The listing builds one solid part. Answer for the finished solid, in the listing's coordinates (mm). A direction names the side the tool comes from. Coordinates: 2 decimals unless noted, no trailing zeros. Order: outer loops, then holes, each group sorted by start corner. A loop starts at its lowest first (then second) coordinate and runs counter-clockwise, first axis right, second up.
from build123d import *

# Parameters (mm, degrees)
EXTRUDE_2_DEPTH      = 10
SKETCH_6_R           = 2.5
CUT_EXTRUDE_1_DEPTH  = 8
SKETCH_7_R           = 5.5
CUT_EXTRUDE_2_DEPTH  = 114.578166916
CUT_EXTRUDE_3_DEPTH  = 114.578166916
CUT_EXTRUDE_4_DEPTH  = 3
FILLET_1_R           = 2
CUT_EXTRUDE_7_DEPTH  = 114.578166916
SKETCH_16_R          = 3.5
CUT_EXTRUDE_8_DEPTH  = 3
SKETCH_18_R          = 2.1
CUT_EXTRUDE_9_DEPTH  = 114.578166916
FILLET_2_R           = 20
FILLET_3_R           = 2.5
SKETCH_20_R          = 3.75
CUT_EXTRUDE_11_DEPTH = 3
SKETCH_21_R          = 2.25
CUT_EXTRUDE_12_DEPTH = 114.578166916
SKETCH_22_R          = 7.1
CUT_EXTRUDE_13_DEPTH = 114.578166916


with BuildPart() as part:
    # 草图5 → 凸台-拉伸2 (new body)
    with BuildSketch(Plane.XY):
        with BuildLine():
            Line((-67.5, 42.938910093), (67.5, 42.938910093))
            ThreePointArc((67.5, 42.938910093), (0, -80), (-67.5, 42.938910093))
        make_face()
    extrude(amount=EXTRUDE_2_DEPTH)

    # 草图6 → 切除-拉伸1 (cut)
    with BuildSketch(Plane(origin=(0, 0, 0), x_dir=(-1, 0, 0), z_dir=(0, 0, -1))):
        with Locations(Location((-51.961524227, 30, 0), (0, 0, 180))):
            Circle(SKETCH_6_R)
        with Locations((-51.961524227, -30)):
            Circle(SKETCH_6_R)
        with Locations((51.961524227, -30)):
            Circle(SKETCH_6_R)
        with Locations(Location((51.961524227, 30, 0), (0, 0, 180))):
            Circle(SKETCH_6_R)
    extrude(amount=-CUT_EXTRUDE_1_DEPTH, mode=Mode.SUBTRACT)

    # 草图7 → 切除-拉伸2 (cut, through all)
    with BuildSketch(Plane(origin=(0, 0, 0), x_dir=(-1, 0, 0), z_dir=(0, 0, -1))):
        with Locations((32.939911054, -27.639867217)):
            Circle(SKETCH_7_R)
        with Locations((32.939911054, 27.639867217)):
            Circle(SKETCH_7_R)
        with Locations((-32.946514438, 27.631995701)):
            Circle(SKETCH_7_R)
        with Locations((-32.946514438, -27.631995701)):
            Circle(SKETCH_7_R)
    extrude(amount=-CUT_EXTRUDE_2_DEPTH, mode=Mode.SUBTRACT)

    # 草图8 → 切除-拉伸3 (cut, through all)
    with BuildSketch(Plane.XY.offset(10)):
        with BuildLine():
            ThreePointArc((-9.2723103, -65.975915967), (0, -66.624299065), (9.2723103, -65.975915967))
            ThreePointArc((9.2723103, -65.975915967), (14.814767997, -58.620826181), (7.459678211, -53.078368485))
            ThreePointArc((7.459678211, -53.078368485), (0, -53.6), (-7.459678211, -53.078368485))
            ThreePointArc((-7.459678211, -53.078368485), (-14.814767997, -58.620826181), (-9.2723103, -65.975915967))
        make_face()
    extrude(amount=-CUT_EXTRUDE_3_DEPTH, mode=Mode.SUBTRACT)

    # 草图9 → 切除-拉伸4 (cut)
    with BuildSketch(Plane.XY.offset(10)):
        with BuildLine():
            Line((-35.246116648, 34.895820279), (-25.683957992, 25.333661623))
            ThreePointArc((-25.683957992, 25.333661623), (-25.683957992, 20.383914155), (-30.63370546, 20.383914155))
            Line((-30.63370546, 20.383914155), (-40.195864116, 29.94607281))
            ThreePointArc((-40.195864116, 29.94607281), (-40.195864116, 34.895820279), (-35.246116648, 34.895820279))
        make_face()
        with BuildLine():
            Line((39.832192061, 29.567925856), (31.010584282, 20.746318078))
            ThreePointArc((31.010584282, 20.746318078), (26.060836814, 20.746318078), (26.060836814, 25.696065546))
            Line((26.060836814, 25.696065546), (34.882444593, 34.517673324))
            ThreePointArc((34.882444593, 34.517673324), (39.832192061, 34.517673324), (39.832192061, 29.567925856))
        make_face()
        with BuildLine():
            Line((-35.246116648, -34.895820279), (-25.683957992, -25.333661623))
            ThreePointArc((-25.683957992, -25.333661623), (-25.683957992, -20.383914155), (-30.63370546, -20.383914155))
            Line((-30.63370546, -20.383914155), (-40.195864116, -29.94607281))
            ThreePointArc((-40.195864116, -29.94607281), (-40.195864116, -34.895820279), (-35.246116648, -34.895820279))
        make_face()
        with BuildLine():
            Line((39.832192061, -29.567925856), (31.010584282, -20.746318078))
            ThreePointArc((31.010584282, -20.746318078), (26.060836814, -20.746318078), (26.060836814, -25.696065546))
            Line((26.060836814, -25.696065546), (34.882444593, -34.517673324))
            ThreePointArc((34.882444593, -34.517673324), (39.832192061, -34.517673324), (39.832192061, -29.567925856))
        make_face()
    extrude(amount=-CUT_EXTRUDE_4_DEPTH, mode=Mode.SUBTRACT)

    # 圆角1
    # the kernel refuses this fillet: 2 mm, written as the material it takes off along each edge
    with BuildSketch(Plane(origin=(32.421388172, -22.157121967, 12.140947066), x_dir=(0.9995822889813627, 0.028900649729367227, 0), z_dir=(0, 0, -1)), Plane(origin=(33.471640703, -33.106869435, 12.140947066), x_dir=(-0.9995822889813627, -0.028900649729367227, 0), z_dir=(0, 0, -1)), Plane(origin=(38.421388172, 28.157121967, 12.140947066), x_dir=(0.028900649729366526, -0.9995822889813627, 0), z_dir=(0, 0, -1)), Plane(origin=(27.471640703, 27.106869435, 12.140947066), x_dir=(-0.028900649729366384, 0.9995822889813627, 0), z_dir=(0, 0, -1)), Plane(origin=(-33.46503732, 33.114740951, 12.140947066), x_dir=(0.9995822889813627, 0.028900649729368344, 0), z_dir=(0, 0, -1)), Plane(origin=(-32.414784788, 22.164993482, 12.140947066), x_dir=(-0.9995822889813627, -0.028900649729368344, 0), z_dir=(0, 0, -1)), Plane(origin=(-27.46503732, -27.114740951, 12.140947066), x_dir=(0.028900649729362526, -0.9995822889813628, 0), z_dir=(0, 0, -1)), Plane(origin=(-38.414784788, -28.164993482, 12.140947066), x_dir=(-0.028900649729357547, 0.9995822889813629, 0), z_dir=(0, 0, -1))) as fillet_1_piece_1:
        with BuildLine():
            CenterArc((0.866697016, -1.995550294), FILLET_1_R, 93.822687788, 42.833428066)
            Line((-0.587797505, -0.622799155), (0, 0))
            ThreePointArc((0, 0), (0.366679507, -0.012236691), (0.733359013, 0))
        make_face()
    extrude(amount=5.140947066, mode=Mode.SUBTRACT)
    with BuildSketch(Plane(origin=(27.471640703, -27.106869435, 12.140947066), x_dir=(-0.028900649729367366, -0.9995822889813627, 0), z_dir=(0, 0, -1)), Plane(origin=(38.421388172, -28.157121967, 12.140947066), x_dir=(0.028900649729367924, 0.9995822889813627, 0), z_dir=(0, 0, -1)), Plane(origin=(33.471640703, 33.106869435, 12.140947066), x_dir=(-0.9995822889813627, 0.028900649729367227, 0), z_dir=(0, 0, -1)), Plane(origin=(32.421388172, 22.157121967, 12.140947066), x_dir=(0.9995822889813627, -0.028900649729367227, 0), z_dir=(0, 0, -1)), Plane(origin=(-38.414784788, 28.164993482, 12.140947066), x_dir=(-0.028900649729367647, -0.9995822889813627, 0), z_dir=(0, 0, -1)), Plane(origin=(-27.46503732, 27.114740951, 12.140947066), x_dir=(0.028900649729362664, 0.9995822889813628, 0), z_dir=(0, 0, -1)), Plane(origin=(-32.414784788, -22.164993482, 12.140947066), x_dir=(-0.9995822889813627, 0.028900649729368066, 0), z_dir=(0, 0, -1)), Plane(origin=(-33.46503732, -33.114740951, 12.140947066), x_dir=(0.9995822889813627, -0.028900649729367785, 0), z_dir=(0, 0, -1))) as fillet_1_piece_2:
        with BuildLine():
            CenterArc((0.866697016, 1.995550294), FILLET_1_R, 223.343884146, 42.833428066)
            Line((-0.587797505, 0.622799155), (0, 0))
            ThreePointArc((0, 0), (0.366679507, 0.012236691), (0.733359013, 0))
        make_face()
    extrude(amount=5.140947066, mode=Mode.SUBTRACT)

    # 草图13 → 切除-拉伸7 (cut, through all)
    with BuildSketch(Plane.XY.offset(10)):
        with BuildLine():
            Line((-31, -40.5), (-64.208177049, -40.5))
            Line((-64.208177049, -40.5), (-68.990941434, -40.5))
            ThreePointArc((-68.990941434, -40.5), (-52.687101579, -60.200243581), (-31, -73.74957627))
            Line((-31, -73.74957627), (-31, -40.5))
        make_face()
        with BuildLine():
            Line((31, -40.5), (31, -73.74957627))
            ThreePointArc((31, -73.74957627), (52.687101579, -60.200243581), (68.990941434, -40.5))
            Line((68.990941434, -40.5), (31, -40.5))
        make_face()
    extrude(amount=-CUT_EXTRUDE_7_DEPTH, mode=Mode.SUBTRACT)

    # 草图16 → 切除-拉伸8 (cut)
    with BuildSketch(Plane(origin=(0, 0, 0), x_dir=(-1, 0, 0), z_dir=(0, 0, -1))):
        with Locations((60, 36.938910093)):
            Circle(SKETCH_16_R)
        with Locations((60, 22.238910093)):
            Circle(SKETCH_16_R)
        with Locations((60, -19.761089907)):
            Circle(SKETCH_16_R)
        with Locations((60, -30.461089907)):
            Circle(SKETCH_16_R)
    cut_extrude_8 = extrude(amount=-CUT_EXTRUDE_8_DEPTH, mode=Mode.SUBTRACT)

    # 草图18 → 切除-拉伸9 (cut, through all)
    with BuildSketch(Plane(origin=(0, 0, 0), x_dir=(-1, 0, 0), z_dir=(0, 0, -1))):
        with Locations((60, -30.461089907)):
            Circle(SKETCH_18_R)
        with Locations((60, -19.761089907)):
            Circle(SKETCH_18_R)
        with Locations((60, 22.238910093)):
            Circle(SKETCH_18_R)
        with Locations((60, 36.938910093)):
            Circle(SKETCH_18_R)
    cut_extrude_9 = extrude(amount=-CUT_EXTRUDE_9_DEPTH, mode=Mode.SUBTRACT)

    # 镜向1: 切除-拉伸8, 切除-拉伸9 across plane
    add(cut_extrude_8.mirror(Plane(origin=(0, 0, 0), x_dir=(0, 0, 1), z_dir=(1, 0, 0))), mode=Mode.SUBTRACT)
    add(cut_extrude_9.mirror(Plane(origin=(0, 0, 0), x_dir=(0, 0, 1), z_dir=(1, 0, 0))), mode=Mode.SUBTRACT)

    # 圆角2
    fillet_2_edges = [part.edges().sort_by_distance(p)[0] for p in [
        (-31, -40.5, 5),
        (31, -40.5, 5),
    ]]
    fillet(fillet_2_edges, radius=FILLET_2_R)

    # 圆角3
    fillet_3_edges = [part.edges().sort_by_distance(p)[0] for p in [
        (-68.990941434, -40.5, 5),
        (68.990941434, -40.5, 5),
    ]]
    fillet(fillet_3_edges, radius=FILLET_3_R)

    # 草图20 → 切除-拉伸11 (cut)
    with BuildSketch(Plane(origin=(0, 0, 0), x_dir=(-1, 0, 0), z_dir=(0, 0, -1))):
        with Locations((23.5, -67.74957627)):
            Circle(SKETCH_20_R)
        with Locations((23.5, -49.74957627)):
            Circle(SKETCH_20_R)
    cut_extrude_11 = extrude(amount=-CUT_EXTRUDE_11_DEPTH, mode=Mode.SUBTRACT)

    # 草图21 → 切除-拉伸12 (cut, through all)
    with BuildSketch(Plane(origin=(0, 0, 0), x_dir=(-1, 0, 0), z_dir=(0, 0, -1))):
        with Locations((23.5, -49.74957627)):
            Circle(SKETCH_21_R)
        with Locations((23.5, -67.74957627)):
            Circle(SKETCH_21_R)
    cut_extrude_12 = extrude(amount=-CUT_EXTRUDE_12_DEPTH, mode=Mode.SUBTRACT)

    # 镜向2: 切除-拉伸11, 切除-拉伸12 across plane
    add(cut_extrude_11.mirror(Plane(origin=(0, 0, 0), x_dir=(0, 0, 1), z_dir=(1, 0, 0))), mode=Mode.SUBTRACT)
    add(cut_extrude_12.mirror(Plane(origin=(0, 0, 0), x_dir=(0, 0, 1), z_dir=(1, 0, 0))), mode=Mode.SUBTRACT)

    # 草图22 → 切除-拉伸13 (cut, through all)
    with BuildSketch(Plane(origin=(0, 0, 0), x_dir=(-1, 0, 0), z_dir=(0, 0, -1))):
        Circle(SKETCH_22_R)
    extrude(amount=-CUT_EXTRUDE_13_DEPTH, mode=Mode.SUBTRACT)


solid = part.part
(1) Given pin 1 Ø4 at (x, y) = (-52.5, 29.5) entering from -Z; pin 2 Ø4 at (y, z) = (-7, 3.5) entering from -X; pin 3 Ø5 at (x, z) = (-38, 6) entering from -Y; pin 4 Ø1.5 at (x, z) = (17.5, 1.5) entering from -Y, each flat-ended and moving along its own axis, determine where each tip first touches the part or whether it passes through.
(2) Find section B-B on y = 0. Determine the outline of the cut face in (x, z), then the cut area to 3 significant figures.
(3) Find section A-A on x = 0. Determine the outline of the cut face in (y, z), then the cut area to 3 significant figures.
(4) The mould has two halves that part along X. Classify faces 1 (the cylindrical face through (-61.94, -20.57, 6.45)), 2 (the flat face through (1, -18, 0)): pulls with the +X half, pulls with the -X half, needs draft (parallel to the pull), parting line crosses it, or undercut.
(5) Find the intervals of material crossed by probe 1 along Y at (x, z) = (52, 4.75); probe 2 along Y at (x, z) = (60, 1.2); probe 3 along X at (y, z) = (-20, 9.25), in increasing order.
(6) A tool of negligible diameter and unlimited length cuts with its end or side. For faces 3 (the flat face through (38, 32, 7)), 4 (the flat face through (52, -30, 8)), 5 (the cylindrical face through (23.012, -69.946, 6.451)), 6 (the flat face through (59, -40.5, 5)), from which of +Z, -Z, +X, -X, +Y, -Y can it reach the whole face along a straight path? Write none if from no direction.
(7) Find section C-C on x = 60. Count the separate pieces of the cut face and the enclosed holes in it, then the cut area to 3 significant figures.
Resolved:
1. pin 1: stops at z = 0
1. pin 2: stops at x = -79.84
1. pin 3: stops at y = -47.86
1. pin 4: stops at y = -78.23
2. outline: (-80, 0) - (-7.1, 0) - (-7.1, 10) - (-80, 10) - close; (7.1, 0) - (80, 0) - (80, 10) - (7.1, 10) - close
2. area: 1,460 mm2
3. outline: (-80, 0) - (-66.62, 0) - (-66.62, 10) - (-80, 10) - close; (-53.6, 0) - (-7.1, 0) - (-7.1, 10) - (-53.6, 10) - close; (7.1, 0) - (42.94, 0) - (42.94, 10) - (7.1, 10) - close
3. area: 957 mm2
4. face 1: undercut
4. face 2: needs draft
5. probe 1: y = -40.5 to -32.5, -27.5 to 27.5, 32.5 to 42.94
5. probe 2: y = -40.5 to -33.96, -26.96 to -23.26, -16.26 to 18.74, 25.74 to 33.44, 40.44 to 42.94
5. probe 3: x = -77.46 to -62.09, -57.91 to -30.18, -26.14 to 27.17, 29.9 to 57.91, 62.09 to 77.46
6. face 3: +Z
6. face 4: -Z
6. face 5: +Z, -Z
6. face 6: +Z, -Z, +X, -Y
7. separate pieces: 5
7. enclosed holes: 0
7. area: 633 mm2
